from build123d import *
from OCP.BRepFilletAPI import BRepFilletAPI_MakeChamfer

# Parameters (mm, degrees)
SKETCH_1_W          = 56
SKETCH_1_H          = 56
EXTRUDE_1_DEPTH     = 12
SKETCH_2_W          = 36
SKETCH_2_H          = 52
CUT_EXTRUDE_1_DEPTH = 10
SKETCH_4_W          = 7
SKETCH_4_H          = 7
EXTRUDE_3_DEPTH     = 3
SKETCH_5_R          = 1.4
CUT_EXTRUDE_3_DEPTH = 8
SKETCH_6_R          = 2.25
CUT_EXTRUDE_4_DEPTH = 42.376321731
SKETCH_7_R          = 4.25
CUT_EXTRUDE_5_DEPTH = 9
CHAMFER_1_SIZE      = 1.5
CHAMFER_1_SIZE_2    = 2
SKETCH_8_R          = 1.4
CUT_EXTRUDE_6_DEPTH = 8


with BuildPart() as part:
    # Эскиз1 → Бобышка-Вытянуть1 (new body)
    with BuildSketch(Plane(origin=(0, 0, 0), x_dir=(1, 0, 0), z_dir=(0, 1, 0))):
        Rectangle(SKETCH_1_W, SKETCH_1_H)
    extrude(amount=EXTRUDE_1_DEPTH)

    # Эскиз2 → Вырез-Вытянуть1 (cut)
    with BuildSketch(Plane(origin=(0, 12, 0), x_dir=(1, 0, 0), z_dir=(0, 1, 0))):
        Rectangle(SKETCH_2_W, SKETCH_2_H)
    extrude(amount=-CUT_EXTRUDE_1_DEPTH, mode=Mode.SUBTRACT)

    # Эскиз4 → Бобышка-Вытянуть3 (add)
    with BuildSketch(Plane(origin=(0, 12, 0), x_dir=(1, 0, 0), z_dir=(0, 1, 0))):
        with Locations((-21.5, -11.5)):
            Rectangle(SKETCH_4_W, SKETCH_4_H)
        with Locations((21.5, 11.5)):
            Rectangle(SKETCH_4_W, SKETCH_4_H)
    extrude(amount=EXTRUDE_3_DEPTH)

    # Эскиз5 → Вырез-Вытянуть3 (cut)
    with BuildSketch(Plane(origin=(0, 15, 0), x_dir=(1, 0, 0), z_dir=(0, 1, 0))):
        with Locations(Location((-21.5, -11.5, 0), (0, 0, 270))):
            Circle(SKETCH_5_R)
        with Locations(Location((21.5, 11.5, 0), (0, 0, 270))):
            Circle(SKETCH_5_R)
    extrude(amount=-CUT_EXTRUDE_3_DEPTH, mode=Mode.SUBTRACT)

    # Эскиз6 → Вырез-Вытянуть4 (cut, through all)
    with BuildSketch(Plane(origin=(0, 12, 0), x_dir=(1, 0, 0), z_dir=(0, 1, 0))):
        with Locations(Location((-23, 19, 0), (0, 0, 270))):
            Circle(SKETCH_6_R)
        with Locations(Location((23, -19, 0), (0, 0, 270))):
            Circle(SKETCH_6_R)
    extrude(amount=-CUT_EXTRUDE_4_DEPTH, mode=Mode.SUBTRACT)

    # Эскиз7 → Вырез-Вытянуть5 (cut)
    with BuildSketch(Plane(origin=(0, 12, 0), x_dir=(1, 0, 0), z_dir=(0, 1, 0))):
        with Locations(Location((-23, 19, 0), (0, 0, 270))):
            Circle(SKETCH_7_R)
        with Locations(Location((23, -19, 0), (0, 0, 270))):
            Circle(SKETCH_7_R)
    extrude(amount=-CUT_EXTRUDE_5_DEPTH, mode=Mode.SUBTRACT)

    # Фаска1
    chamfer_1_edges_1 = [part.edges().sort_by_distance(p)[0] for p in [
        (-23, 3, -21.25),
    ]]
    chamfer_1_side_1 = [part.faces().sort_by_distance(p)[0] for p in [
        (-23, 2.97, -21.25),
    ]]
    chamfer_1_edges_2 = [part.edges().sort_by_distance(p)[0] for p in [
        (23, 3, 16.75),
    ]]
    chamfer_1_side_2 = [part.faces().sort_by_distance(p)[0] for p in [
        (23, 2.97, 16.75),
    ]]
    chamfer_1 = BRepFilletAPI_MakeChamfer(part.part.solid().wrapped)
    for e in chamfer_1_edges_1:
        chamfer_1.Add(CHAMFER_1_SIZE - 0.0001, CHAMFER_1_SIZE_2 - 0.0001, e.wrapped, chamfer_1_side_1[0].wrapped)
    for e in chamfer_1_edges_2:
        chamfer_1.Add(CHAMFER_1_SIZE - 0.0001, CHAMFER_1_SIZE_2 - 0.0001, e.wrapped, chamfer_1_side_2[0].wrapped)
    add(Compound.cast(chamfer_1.Shape()), mode=Mode.REPLACE)  # a hair under: the kernel refuses the full size

    # Эскиз8 → Вырез-Вытянуть6 (cut)
    with BuildSketch(Plane(origin=(0, 12, 0), x_dir=(1, 0, 0), z_dir=(0, 1, 0))):
        with Locations(Location((-25, 25, 0), (0, 0, 270))):
            Circle(SKETCH_8_R)
        with Locations(Location((25, -25, 0), (0, 0, 270))):
            Circle(SKETCH_8_R)
        with Locations(Location((-25, -25, 0), (0, 0, 270))):
            Circle(SKETCH_8_R)
        with Locations(Location((25, 25, 0), (0, 0, 270))):
            Circle(SKETCH_8_R)
    extrude(amount=-CUT_EXTRUDE_6_DEPTH, mode=Mode.SUBTRACT)


solid = part.part
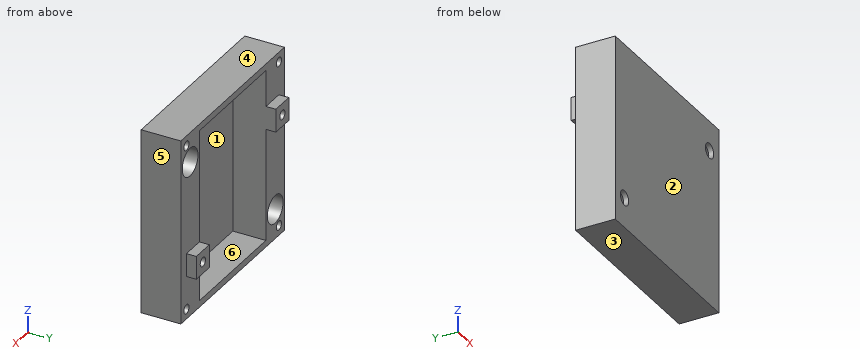
Verification items for the finished model (mm, model axes). Face numbers are marked on the shaded views. A direction names the side the tool comes from. Give positions to 0.01 mm unless a question says otherwise; leave off trailing zeros. Write each loop counter-clockwise with the first axis right and the second up, starting at its lowest first coordinate (ties: lowest second). Pieces come first, ordered by that corner, then holes. Notation, with made-up numbers: M 50.5,39 L 84.5,39 A23 cw 84.5,59 Z; hole C 22,1 d4. An arc over 180 degrees is marked long. Use CSV: the item, a comma, the result in double quotes.
1) Material ranges on line 1 along X through (y, z) = (8.25, 25); line 2 along Z through (x, y) = (-5, 8.5); line 3 along X through (y, z) = (8.5, 5), recorded low to high.
Final values:
line 1,"-28 to -26.4, -23.6 to -18, 18 to 23.6, 26.4 to 28"
line 2,"-28 to -26, 26 to 28"
line 3,"-28 to -18, 18 to 28"
2) Access from +Z, -Z, +X, -X, +Y, -Y to the whole of each face (thin tool, end or side, straight path). Record for the marked faces 5 and 6.
Final values:
face 5,"+Z, -Z, +X, +Y, -Y"
face 6,"+Y"
3) Cross-section at D-D (x = 16.5). Enter the section's corners in (y, z), plus the area to 3 significant figures.
Final values:
outline,"M 0,-28 L 12,-28 L 12,-26 L 2,-26 L 2,26 L 12,26 L 12,28 L 0,28 Z"
area,"152 mm²"
4) Cross-section at A-A (y = 13.25). Enter the section's corners in (x, z).
Final values:
outline,"M -25,8 L -18,8 L -18,15 L -25,15 Z; M 18,-15 L 25,-15 L 25,-8 L 18,-8 Z; hole C -21.5,11.5 d2.8; hole C 21.5,-11.5 d2.8"
5) Go/stop test with flat-tipped pins: pin 1 Ø2 at (x, z) = (24.5, -24.5) entering from +Y; pin 2 Ø11 at (x, z) = (-0.5, 2) entering from +Y; pin 3 Ø3.5 at (x, y) = (20.5, 14) entering from +Z. Record where each tip stops, or that it passes through.
Final values:
pin 1,"y = 12"
pin 2,"y = 2"
pin 3,"z = -8"
6) Release check for a two-part mould opening along Z. For the marked faces 1, 2, 3 and 4 record: released by +Z, released by -Z, zero draft, split by the parting line, or undercut.
Final values:
face 1,"undercut"
face 2,"zero draft"
face 3,"released by -Z"
face 4,"released by +Z"
7) Cross-section at B-B (z = 11.5). Enter the section's corners in (x, y), plus the area to 3 significant figures.
Final values:
outline,"M -28,0 L 28,0 L 28,12 L 18,12 L 18,2 L -18,2 L -18,15 L -20.1,15 L -20.1,7 L -22.9,7 L -22.9,15 L -25,15 L -25,12 L -28,12 Z"
area,"311 mm²"
